from build123d import *

# Parameters (mm, degrees)
F0_R     = 4
F1_DEPTH = 1


with BuildPart() as f1:
    # F0 (on Front) → F1 (new body)
    with BuildSketch(Plane.XZ):
        with BuildLine():
            ThreePointArc((-42.428788, 22.197763), (-22.393428, 40.636528), (0.736568, 26.269656))
            Line((0.736568, 26.269656), (7.82161, 7.734496))
            Line((7.82161, 7.734496), (445.831745, 440.866256))
            Line((445.831745, 440.866256), (409.571118, 551.809463))
            ThreePointArc((409.571118, 551.809463), (403.393924, 553.012383), (397.791506, 555.879027))
            Line((397.791506, 555.879027), (-153.711431, 555.879027))
            Line((-153.711431, 555.879027), (-163.711431, 555.879027))
            Line((-163.711431, 555.879027), (-176.433934, 530.299822))
            Line((-176.433934, 530.299822), (-292.672837, 296.595913))
            Line((-292.672837, 296.595913), (-429.805557, 108.635613))
            ThreePointArc((-429.805557, 108.635613), (-433.055197, 105.145969), (-437.038546, 102.524765))
            Line((-437.038546, 102.524765), (-467.979575, 87.098137))
            ThreePointArc((-467.979575, 87.098137), (-479.031049, 77.063624), (-483.216559, 62.73505))
            Line((-483.216559, 62.73505), (-444.218322, 62.364245))
            ThreePointArc((-444.218322, 62.364245), (-439.992581, 60.566627), (-438.27564, 56.307469))
            ThreePointArc((-438.27564, 56.307469), (-440.073258, 52.081729), (-444.332415, 50.364787))
            Line((-444.332415, 50.364787), (-483.330653, 50.735592))
            Line((-483.330653, 50.735592), (-473.742625, 39.200006))
            ThreePointArc((-473.742625, 39.200006), (-462.016917, 29.862605), (-447.542263, 25.968544))
            Line((-447.542263, 25.968544), (-119.640526, 6.942116))
            ThreePointArc((-119.640526, 6.942116), (-119.539343, 30.38703), (-113.982147, 53.164032))
            ThreePointArc((-113.982147, 53.164032), (-112.028876, 55.605369), (-109.00742, 56.409233))
            Line((-109.00742, 56.409233), (-91.138541, 55.372396))
            ThreePointArc((-91.138541, 55.372396), (-94.609764, 47.818656), (-97.278364, 39.945477))
            ThreePointArc((-97.278364, 39.945477), (-100.140537, 22.963258), (-99.30184, 5.761968))
            Line((-99.30184, 5.761968), (-45.922757, 2.664658))
            Line((-45.922757, 2.664658), (-42.428788, 22.197763))
        make_face()
        with BuildLine():
            ThreePointArc((-219.185589, 82.205842), (-234.185589, 97.205842), (-219.185589, 112.205842))
            Line((-219.185589, 112.205842), (-139.185589, 112.205842))
            ThreePointArc((-139.185589, 112.205842), (-124.185589, 97.205842), (-139.185589, 82.205842))
            Line((-139.185589, 82.205842), (-219.185589, 82.205842))
        make_face(mode=Mode.SUBTRACT)
        with BuildLine():
            ThreePointArc((-238.884885, 257.620199), (-269.539195, 249.087128), (-278.072266, 279.741438))
            Line((-278.072266, 279.741438), (-223.998126, 375.532812))
            ThreePointArc((-223.998126, 375.532812), (-193.343817, 384.065883), (-184.810746, 353.411573))
            Line((-184.810746, 353.411573), (-238.884885, 257.620199))
        make_face(mode=Mode.SUBTRACT)
        with Locations((-83.001788, 494.079027)):
            Circle(F0_R, mode=Mode.SUBTRACT)
        with Locations((9.507399, 72.687717)):
            Circle(F0_R, mode=Mode.SUBTRACT)
        with Locations((386.357424, 494.079027)):
            Circle(F0_R, mode=Mode.SUBTRACT)
        with BuildLine():
            ThreePointArc((-109.00742, 56.409233), (-99.197738, 50.987949), (-97.278364, 39.945477))
            ThreePointArc((-97.278364, 39.945477), (-94.609764, 47.818656), (-91.138541, 55.372396))
            Line((-91.138541, 55.372396), (-109.00742, 56.409233))
        make_face()
        with BuildLine():
            Line((-153.711431, 555.879027), (397.791506, 555.879027))
            ThreePointArc((397.791506, 555.879027), (388.241023, 574.279027), (397.791506, 592.679027))
            Line((397.791506, 592.679027), (-153.711431, 592.679027))
            ThreePointArc((-153.711431, 592.679027), (-135.311431, 574.279027), (-153.711431, 555.879027))
        make_face()
        with BuildLine():
            Line((-153.711431, 592.679027), (397.791506, 592.679027))
            ThreePointArc((397.791506, 592.679027), (403.393924, 595.545671), (409.571118, 596.748591))
            Line((409.571118, 596.748591), (418.046209, 622.679027))
            Line((418.046209, 622.679027), (406.046209, 622.679027))
            ThreePointArc((406.046209, 622.679027), (403.924889, 623.557707), (403.046209, 625.679027))
            ThreePointArc((403.046209, 625.679027), (403.924889, 627.800347), (406.046209, 628.679027))
            Line((406.046209, 628.679027), (420.007247, 628.679027))
            Line((420.007247, 628.679027), (445.831745, 707.691799))
            Line((445.831745, 707.691799), (7.82161, 1140.823559))
            Line((7.82161, 1140.823559), (0.736568, 1122.288398))
            ThreePointArc((0.736568, 1122.288398), (-22.393428, 1107.921526), (-42.428788, 1126.360291))
            Line((-42.428788, 1126.360291), (-45.922757, 1145.893396))
            Line((-45.922757, 1145.893396), (-447.542263, 1122.58951))
            ThreePointArc((-447.542263, 1122.58951), (-462.016917, 1118.695449), (-473.742625, 1109.358048))
            Line((-473.742625, 1109.358048), (-483.330653, 1097.822462))
            Line((-483.330653, 1097.822462), (-444.332415, 1098.193267))
            ThreePointArc((-444.332415, 1098.193267), (-440.073258, 1096.476326), (-438.27564, 1092.250585))
            ThreePointArc((-438.27564, 1092.250585), (-439.992581, 1087.991428), (-444.218322, 1086.19381))
            Line((-444.218322, 1086.19381), (-483.216559, 1085.823005))
            ThreePointArc((-483.216559, 1085.823005), (-479.031049, 1071.494431), (-467.979575, 1061.459917))
            Line((-467.979575, 1061.459917), (-437.038546, 1046.033289))
            ThreePointArc((-437.038546, 1046.033289), (-433.055197, 1043.412085), (-429.805557, 1039.922441))
            Line((-429.805557, 1039.922441), (-292.672837, 851.962142))
            Line((-292.672837, 851.962142), (-178.632735, 622.679027))
            Line((-178.632735, 622.679027), (-176.433934, 618.258232))
            Line((-176.433934, 618.258232), (-163.711431, 592.679027))
            Line((-163.711431, 592.679027), (-153.711431, 592.679027))
        make_face()
        with Locations((-83.001788, 654.479027)):
            Circle(F0_R, mode=Mode.SUBTRACT)
        with BuildLine():
            ThreePointArc((-281.759139, 875.347847), (-276.070425, 895.784053), (-255.634219, 890.095339))
            Line((-255.634219, 890.095339), (-194.186333, 781.241505))
            ThreePointArc((-194.186333, 781.241505), (-199.875047, 760.805298), (-220.311253, 766.494012))
            Line((-220.311253, 766.494012), (-281.759139, 875.347847))
        make_face(mode=Mode.SUBTRACT)
        with Locations((386.357424, 654.479027)):
            Circle(F0_R, mode=Mode.SUBTRACT)
        with Locations((9.507399, 1075.870338)):
            Circle(F0_R, mode=Mode.SUBTRACT)
    extrude(amount=F1_DEPTH)


solid = f1.part
Model file for the job. Use its own axes, mm. A direction names the side the tool comes from. Coordinates: 2 decimals unless noted, no trailing zeros. Order: outer loops, then holes, each group sorted by start corner. A loop starts at its lowest first (then second) coordinate and runs counter-clockwise, first axis right, second up. Notation, with made-up numbers: (7, 8.5) -> (59, 8.5) arc R22 ccw to (59, 44.5) -> close; hole circle Ø7 at (-11, 72.5). An arc over 180 degrees is marked (long way). Return JSON: item names as keys, results as strings. Group by question number.
Item 1: Saw through at A-A on z = 802.5. Write the cut outline in (x, y).
Item 2: Flat gauge pins, fed straight in: P1, Ø1, axis at x = 202.5, z = 351, coming from the +Y side; P2, Ø0.5, axis at x = -159, y = -0.5, coming from the +Z side. Where does each tip first touch, or does it go through?
Item 3: Saw through at D-D on x = 93. Write the cut outline in (y, z), then the cut area to 3 significant figures.
Item 4: Pull direction Z, two halves, no side cores. Call faces 6 (the flat face through (223.76, -0.49, 221.27)), 7 (the flat face through (-25, 0, 582)), 8 (the flat face through (432.74, -0.49, 667.63)), 9 (the flat face through (-360.3, -0.5, 203.9)): pulls with the +Z half, pulls with the -Z half, needs draft (parallel to the pull), parting line crosses it, or undercut.
Item 5: Wall check: line 1 along Z through (x, y) = (-445, -0.45); line 2 along Z through (x, y) = (-268.5, -0.4); line 3 along X through (y, z) = (-0.3, 374.5). Give the ranges that are in metal, low to high. Write a range as [from, to].
Item 6: Saw through at B-B on z = 341. Write the cut outline in (x, y).
Item 7: Tool access for faces 1 (the flat face through (229.89, -0.49, 921.23)), 2 (the flat face through (-243.921, -0.493, 1134.405)), 3 (the flat face through (-250.605, -0.493, 820.159)), 4 (the flat face through (-362.2, -0.49, 947.26)), 5 (the flat face through (427.955, -0.493, 495.561)): list every direction of +Z, -Z, +X, -X, +Y, -Y with a clear straight run to the whole face (end or side of a thin tool).
Item 8: Saw through at C-C on y = -0.8. State how many separate pieces and enclosed holes the cut face has, then the cut area to 3 significant figures.
Values found:
{
 "1": {"outline": "(-268.07, -1) -> (-240.64, -1) -> (-240.64, 0) -> (-268.07, 0) -> close; (-206.19, -1) -> (349.96, -1) -> (349.96, 0) -> (-206.19, 0) -> close"},
 "2": {"P1": "stops at y = 0", "P2": "stops at z = 1139.35"},
 "3": {"outline": "(-1, 91.96) -> (0, 91.96) -> (0, 1056.59) -> (-1, 1056.59) -> close", "area": "965 mm2"},
 "4": {"face 6": "pulls with the -Z half", "face 7": "needs draft", "face 8": "undercut", "face 9": "undercut"},
 "5": {"line 1": "z = [25.82, 50.37], [62.37, 98.56], [1050, 1086.19], [1098.19, 1122.74]", "line 2": "z = [15.58, 248.54], [296.7, 345.2], [803.36, 851.86], [897.72, 1132.98]", "line 3": "x = [-253.93, -224.58], [-184.26, 378.72]"},
 "6": {"outline": "(-270.59, -1) -> (-243.49, -1) -> (-243.49, 0) -> (-270.59, 0) -> close; (-191.82, -1) -> (344.84, -1) -> (344.84, 0) -> (-191.82, 0) -> close"},
 "7": {"face 1": "+Z, +X, +Y, -Y", "face 2": "+Z, -X, +Y, -Y", "face 3": "+Y, -Y", "face 4": "-X, +Y, -Y", "face 5": "+X, +Y, -Y"},
 "8": {"separate pieces": "1", "enclosed holes": "9", "area": "638,000 mm2"}
}
